Input: part model. Units: mm. Frame: model coordinates. Face numbers are marked on the shaded views. A direction names the side the tool comes from. Round coordinates to 2 decimals unless told otherwise and drop trailing zeros. Loops run counter-clockwise (first coordinate to the right, second up) from the corner with the lowest first, then second, coordinate; pieces in that order, holes last.
1) Section B-B, the plane x = -1. Return loops of the section in (y, z).
2) First-contact query: pin 1 (4.5 mm diameter, centred on y = 11, z = 7.5, fed in from -X); pin 2 (0.8 mm diameter, centred on x = 4.5, z = 12, fed in from -Y); pin 3 (1 mm diameter, centred on x = 8, y = 5, fed in from -Z); pin 4 (5 mm diameter, centred on x = 1.5, z = 17.5, fed in from -Y). Flat tips, straight axial feed; report the tip coordinate or a pass-through.
3) Ray query, line 1 along Z through (x, y) = (-1.3, -22); line 2 along X through (y, z) = (1.5, 15); line 3 along X through (y, z) = (-16, 12.75). Return the intervals inside material, ascending.
4) Access query for the marked faces 4, 5 and 6. Directions: +Z, -Z, +X, -X, +Y, -Y. A direction counts if a zero-diameter tool reaches every point of the face in a straight line with its end or side. Return the directions, or none.
5) Section A-A, the plane z = 7. Return loops of the section in (x, y), and give its area (3 significant figures).
6) Section C-C, the plane z = 10. State how many separate pieces and enclosed holes the cut face has, and give its area (3 significant figures).
7) Draft query along Z for the marked faces 1, 2 and 3. Return one class per face: pulls with the +Z half, pulls with the -Z half, needs draft (parallel to the pull), parting line crosses it, or undercut.
8) Section D-D, the plane y = 9. Return loops of the section in (x, z), and give its area (3 significant figures).
from build123d import *

# Parameters (mm, degrees)
EXTRUDE_1_DEPTH     = 20
SKETCH_2_R          = 1.5
EXTRUDE_2_DEPTH     = 4
FILLET_6_R          = 1
CUT_EXTRUDE_1_REACH = 51.81


with BuildPart() as part:
    # 草图1 → 凸台-拉伸1 (new body)
    with BuildSketch(Plane.XY):
        Polygon((5.8, 6), (3, 6), (3, 3), (5.8, 3), (5.8, 0), (0, 0), (0, -2), (-4, -2), (-4, 3), (0, 14), (20, 14), (20, 0), (14.2, 0), (14.2, 3), (17, 3), (17, 6), (14.2, 6), (14.2, 10), (5.8, 10), align=None)
    extrude(amount=EXTRUDE_1_DEPTH)

    # 草图2 → 凸台-拉伸2 (add)
    with BuildSketch(Plane.ZY.offset(4)):
        with BuildLine():
            Line((5, -2), (15, -2))
            Line((15, -2), (15, -22))
            ThreePointArc((15, -22), (10, -27), (5, -22))
            Line((5, -22), (5, -2))
        make_face()
        with Locations(Location((10, -22, 0), (0, 0, 270))):
            Circle(SKETCH_2_R, mode=Mode.SUBTRACT)
    extrude(amount=-EXTRUDE_2_DEPTH)

    # 圆角6
    fillet_6_edges = [part.edges().sort_by_distance(p)[0] for p in [
        (4.4, 3, 20),
        (3, 4.5, 20),
        (15.6, 3, 0),
        (17, 4.5, 0),
        (15.6, 6, 0),
        (4.4, 6, 0),
        (3, 4.5, 0),
        (4.4, 3, 0),
        (4.4, 6, 20),
        (-4, 3, 10),
        (0, 14, 10),
        (15.6, 6, 20),
        (17, 4.5, 20),
        (15.6, 3, 20),
    ]]
    fillet(fillet_6_edges, radius=FILLET_6_R)

    # 草图3 → 切除-拉伸1 (cut, up to next)
    with BuildSketch(Plane(origin=(0, 14, 0), x_dir=(1, 0, 0), z_dir=(0, 1, 0)), mode=Mode.PRIVATE) as cut_extrude_1_sk1:
        with BuildLine():
            Line((9.150213632, -3), (9.150213632, -17))
            ThreePointArc((9.150213632, -17), (10.650213632, -18.5), (12.150213632, -17))
            Line((12.150213632, -17), (12.150213632, -3))
            ThreePointArc((12.150213632, -3), (10.650213632, -1.5), (9.150213632, -3))
        make_face()
    cut_extrude_1_tool1 = extrude(cut_extrude_1_sk1.sketch, amount=-CUT_EXTRUDE_1_REACH, mode=Mode.PRIVATE) & part.part
    add(cut_extrude_1_tool1.solids().sort_by_distance((10.650214, 14, 10))[0], mode=Mode.SUBTRACT)


solid = part.part
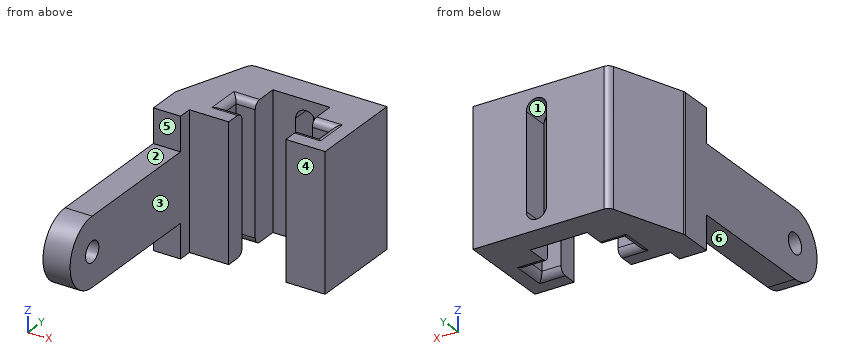
Final values:
1. outline: (-22, 5) - (-2, 5) - (-2, 0) - (11.25, 0) - (11.25, 20) - (-2, 20) - (-2, 15) - (-22, 15) arc R5 ccw to start; hole circle Ø3 at (-22, 10)
2. pin 1: stops at x = -1.91
2. pin 2: stops at y = 0
2. pin 3: passes through
2. pin 4: stops at y = -2
3. line 1: z = 5 to 8.5, 11.5 to 15
3. line 2: x = -4 to 5.8, 14.2 to 20
3. line 3: x = -4 to 0
4. face 4: +Z, -Z, +X, -Y
4. face 5: +Z, +X, -X, -Y
4. face 6: -Z, +X, -X, -Y
5. outline: (-4, -26) - (0, -26) - (0, 0) - (5.8, 0) - (5.8, 3) - (3, 3) - (3, 6) - (5.8, 6) - (5.8, 10) - (9.15, 10) - (9.15, 14) - (0.7, 14) arc R1 ccw to (-0.24, 13.34) - (-3.94, 3.17) arc R1 ccw to (-4, 2.82) - close; (12.15, 10) - (14.2, 10) - (14.2, 6) - (17, 6) - (17, 3) - (14.2, 3) - (14.2, 0) - (20, 0) - (20, 14) - (12.15, 14) - close
5. area: 305 mm2
6. separate pieces: 3
6. enclosed holes: 0
6. area: 297 mm2
7. face 1: undercut
7. face 2: pulls with the +Z half
7. face 3: needs draft
8. outline: (-1.82, 0) - (5.8, 0) - (5.8, 20) - (-1.82, 20) - close; (14.2, 0) - (20, 0) - (20, 20) - (14.2, 20) - close
8. area: 268 mm2
